Check sheet for the modelled part. Datum: model origin and axes. Units: mm. Face numbers are marked on the shaded views. Coordinates: 2 decimals unless noted, no trailing zeros. Loops run counter-clockwise (first coordinate to the right, second up) from the corner with the lowest first, then second, coordinate; pieces in that order, holes last. Notation, with made-up numbers: M -9,86 L 4,86 A20 cw 4,91 Z; hole C -16,55 d11. An arc over 180 degrees is marked long. Use CSV: the item, a comma, the result in double quotes. Start each with the question number.
(1) Section check A-A on y = 0. Record the cut outline in (x, z).
(2) Draft check along X on the marked faces 1, 2 and 3. Enter one of: pulls with the +X half, pulls with the -X half, needs draft (parallel to the pull), parting line crosses it, or undercut.
(3) Section check C-C on x = -20. Record the cut outline in (y, z), and give its area (3 significant figures).
(4) Scan lines: line 1 (Y direction, x = -0.5, z = 4.45); line 2 (Y direction, x = 21, z = 0.45); line 3 (X direction, y = 30.5, z = 2.1). Record each from-to range of solid material in increasing order.
(5) Go/stop test with flat-tipped pins: pin 1 Ø12 at (x, y) = (-16, -16) entering from +Z; pin 2 Ø1 at (x, z) = (-27, 1.5) entering from -Y. Record where each tip stops, or that it passes through.
Autodesk Inventor part; units mm, degrees
ref_plane "YZ Plane" through (0, 0, 0) normal (1, 0, 0) x (0, 1, 0)
ref_plane "XZ Plane" through (0, 0, 0) normal (0, 1, 0) x (-1, 0, 0)
ref_plane "XY Plane" through (0, 0, 0) normal (0, 0, 1) x (1, 0, 0)
sketch "스케치1" plane through (0, 0, 0) normal (0, 0, 1) x (1, 0, 0)
  circle A0 centre (0, 0) radius 44.5
  line L0 (-42, -42) -> (42, -42)
  line L1 (42, -42) -> (42, 42)
  line L2 (42, 42) -> (-42, 42)
  line L3 (-42, 42) -> (-42, -42)
  line L4 (-42, -42) -> (42, 42) construction
  line L5 (42, -42) -> (-42, 42) construction
  circle A1 centre (0, 0) radius 27.5
  point P0 (-42, 14.7054)
  point P1 (-42, -14.7054)
  point P2 (-14.7054, -42)
  point P3 (14.7054, -42)
  point P4 (42, -14.7054)
  point P5 (42, 14.7054)
  point P6 (14.7054, 42)
  point P7 (-14.7054, 42)
  dimension "d0" = 89
  dimension "d1" = 84
  dimension "d2" = 84
  dimension "d3" = 55
extrude "돌출1" add sketch "스케치1" along normal blind 5 contours L1 A0 L0 L3 L2
sketch "스케치4" plane through (0, 0, 5) normal (0, 0, 1) x (1, 0, 0)
  circle A0 centre (0, 35) radius 2 construction
  circle A1 centre (0, 0) radius 33 construction
  circle A2 centre (0, 35) radius 2.15
  dimension "d25" = 4
  dimension "d26" = 66
  dimension "d27" = 4.3
extrude "돌출5" cut sketch "스케치4" against normal blind 10
pattern_circular "원형 패턴3" count 16 over 360 about axis through (0, 0, 0) along (0, 0, 1) of "돌출5"
properties part number "감속기어1 - 하우징 커버"
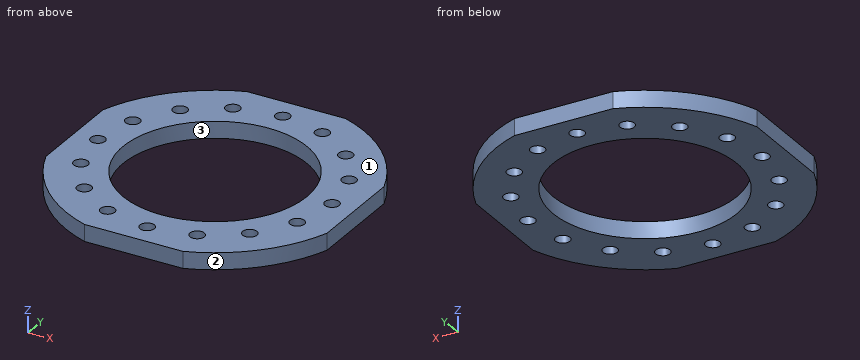
Outcome:
1,outline,"M -42,0 L -37.15,0 L -37.15,5 L -42,5 Z; M -32.85,0 L -27.5,0 L -27.5,5 L -32.85,5 Z; M 27.5,0 L 32.85,0 L 32.85,5 L 27.5,5 Z; M 37.15,0 L 42,0 L 42,5 L 37.15,5 Z"
2,face 1,"needs draft"
2,face 2,"pulls with the +X half"
2,face 3,"undercut"
3,outline,"M -39.75,0 L -18.87,0 L -18.87,5 L -39.75,5 Z; M 18.87,0 L 39.75,0 L 39.75,5 L 18.87,5 Z"
3,area,"209 mm²"
4,line 1,"y = -42 to -37.09, -32.91 to -27.5, 27.5 to 32.91, 37.09 to 42"
4,line 2,"y = -39.23 to -17.76, 17.76 to 39.23"
4,line 3,"x = -32.4 to -14.51, -12.27 to 12.27, 14.51 to 32.4"
5,pin 1,"stops at z = 5"
5,pin 2,"stops at y = -35.75"
